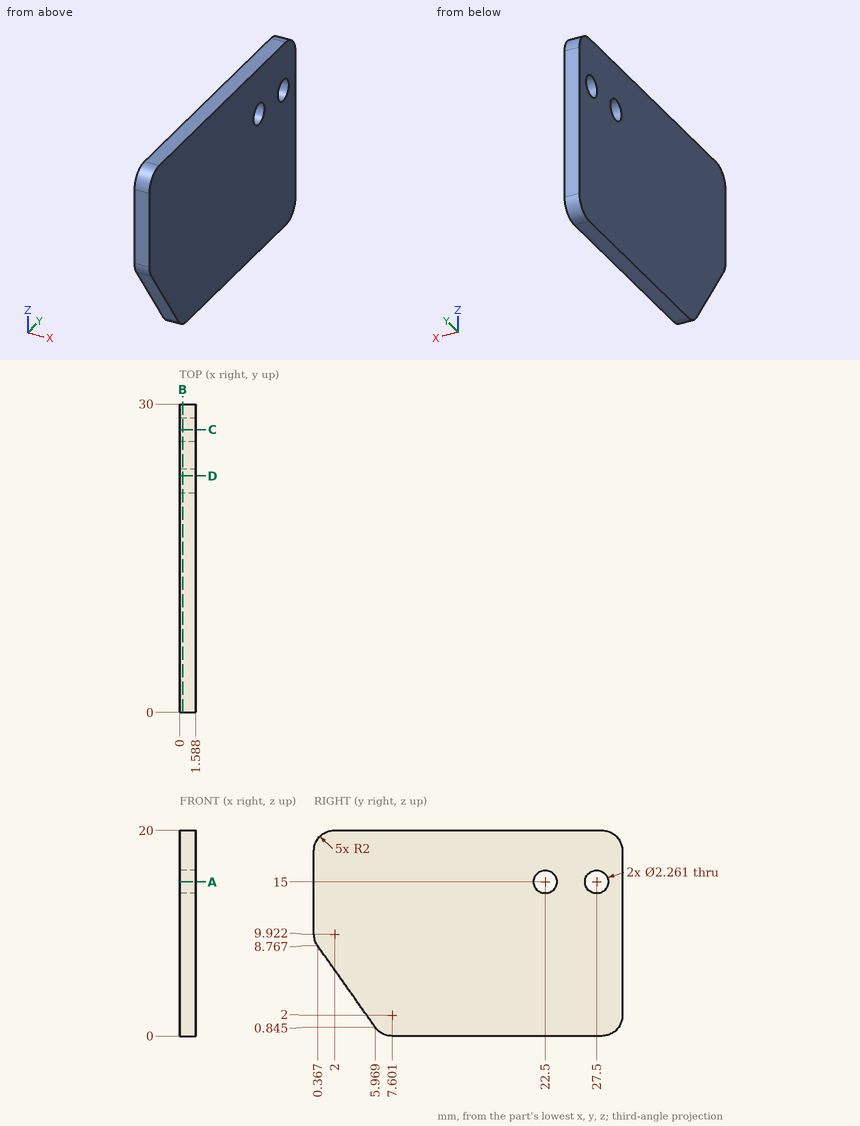
The drawing under review shows one solid part. Ordinate dimensions are in mm from its lowest x, y, z. Coordinates: 2 decimals unless noted, no trailing zeros. Write each loop counter-clockwise with the first axis right and the second up, starting at its lowest first coordinate (ties: lowest second). Pieces come first, ordered by that corner, then holes.
1) Insertion check: pin 1 (2 mm diameter, centred on y = 27.5, z = 15, fed in from -X). The pin has a flat end and moves straight along its axis. Give the tip position at first contact, or say it passes through.
2) Add section A-A (z = 15). Write out the cut boundary in (x, y).
3) Add section D-D (y = 23). Write out the cut boundary in (x, z).
4) To check wall thickness, follow L1, parallel to Z at x = 1.1, y = 27.5; L2, parallel to Z at x = 0.95, y = 26.5 (1 decimal); L3, parallel to Y at x = 1.05, z = 19. State the ranges of each line that lie inside material, in increasing order.
5) Add section B-B (x = 0.3). Write out the cut boundary in (y, z) (1 decimal), plus the area to 3 significant figures.
6) Add section C-C (y = 27.5). Write out the cut boundary in (x, z).
Check result:
1. pin 1: passes through
2. outline: (0, 0) - (1.59, 0) - (1.59, 21.37) - (0, 21.37) - close; (0, 23.63) - (1.59, 23.63) - (1.59, 26.37) - (0, 26.37) - close; (0, 28.63) - (1.59, 28.63) - (1.59, 30) - (0, 30) - close
3. outline: (0, 0) - (1.59, 0) - (1.59, 13.99) - (0, 13.99) - close; (0, 16.01) - (1.59, 16.01) - (1.59, 20) - (0, 20) - close
4. L1: z = 0 to 13.87, 16.13 to 20
4. L2: z = 0 to 14.5, 15.5 to 20
4. L3: y = 0.27 to 29.73
5. outline: (0, 9.9) arc R2 ccw to (0.4, 8.8) - (6, 0.8) arc R2 ccw to (7.6, 0) - (28, 0) arc R2 ccw to (30, 2) - (30, 18) arc R2 ccw to (28, 20) - (2, 20) arc R2 ccw to (0, 18) - close; hole circle Ø2.3 at (22.5, 15); hole circle Ø2.3 at (27.5, 15)
5. area: 559 mm2
6. outline: (0, 0) - (1.59, 0) - (1.59, 13.87) - (0, 13.87) - close; (0, 16.13) - (1.59, 16.13) - (1.59, 20) - (0, 20) - close
